Here's how the part is built. I have some questions about the finished solid (model axes, mm). A direction names the side the tool comes from. Coordinates: 2 decimals unless noted, no trailing zeros. Write each loop counter-clockwise with the first axis right and the second up, starting at its lowest first coordinate (ties: lowest second). Pieces come first, ordered by that corner, then holes.
```python
from build123d import *

# Parameters (mm, degrees)
BOSS_EXTRUDE1_DEPTH = 6.5


with BuildPart() as part:
    # Sketch1 → Boss-Extrude1 (new body)
    with BuildSketch(Plane.XY):
        with BuildLine():
            Line((9.441130989, 75.543158327), (10.978710332, 87.222232942))
            ThreePointArc((10.978710332, 87.222232942), (10.23623569, 89.872312951), (7.807292937, 91.166310537))
            ThreePointArc((7.807292937, 91.166310537), (0, 91.5), (-7.807292937, 91.166310537))
            ThreePointArc((-7.807292937, 91.166310537), (-10.23623569, 89.872312951), (-10.978710332, 87.222232942))
            Line((-10.978710332, 87.222232942), (-9.441130989, 75.543158327))
            ThreePointArc((-9.441130989, 75.543158327), (-8.278784327, 73.368560674), (-5.971073974, 72.5))
            Line((-5.971073974, 72.5), (5.971073974, 72.5))
            ThreePointArc((5.971073974, 72.5), (8.278784327, 73.368560674), (9.441130989, 75.543158327))
        make_face()
        with BuildLine():
            Line((-9.49154304, 87.418022231), (-7.953963697, 75.738947616))
            ThreePointArc((-7.953963697, 75.738947616), (-7.289765605, 74.496320385), (-5.971073974, 74))
            Line((-5.971073974, 74), (5.971073974, 74))
            ThreePointArc((5.971073974, 74), (7.289765605, 74.496320385), (7.953963697, 75.738947616))
            Line((7.953963697, 75.738947616), (9.49154304, 87.418022231))
            ThreePointArc((9.49154304, 87.418022231), (9.067271816, 88.932353664), (7.679304529, 89.671780856))
            ThreePointArc((7.679304529, 89.671780856), (0, 90), (-7.679304529, 89.671780856))
            ThreePointArc((-7.679304529, 89.671780856), (-9.067271816, 88.932353664), (-9.49154304, 87.418022231))
        make_face(mode=Mode.SUBTRACT)
    extrude(amount=BOSS_EXTRUDE1_DEPTH)


solid = part.part
```
1) Imagine slicing it at C-C on z = 1.25. Please give me the cut outline in (x, y), then the cut area to 3 significant figures.
Values follow:
outline: (-10.98, 87.22) - (-9.44, 75.54) arc R3.5 ccw to (-5.97, 72.5) - (5.97, 72.5) arc R3.5 ccw to (9.44, 75.54) - (10.98, 87.22) arc R3.5 ccw to (7.81, 91.17) arc R91.5 ccw to (-7.81, 91.17) arc R3.5 ccw to start; hole (-9.49, 87.42) - (-7.95, 75.74) arc R2 ccw to (-5.97, 74) - (5.97, 74) arc R2 ccw to (7.95, 75.74) - (9.49, 87.42) arc R2 ccw to (7.68, 89.67) arc R90 ccw to (-7.68, 89.67) arc R2 ccw to start
area: 102 mm2
2) We'd pull the mould along X, two halves only. Please class faces 3 (the face through (-0.1, 90.5, 6.5)), 4 (the face through (-10.211, 89.903, 3.204)), 5 (the face through (-8.734, 81.66, 3.204)), 6 (the face through (10.26, 89.84, 3.2)): pulls with the +X half, pulls with the -X half, needs draft (parallel to the pull), parting line crosses it, or undercut.
Values follow:
face 3: needs draft
face 4: pulls with the -X half
face 5: undercut
face 6: pulls with the +X half
3) Imagine slicing it at A-A on x = -6.5. Please give me the cut outline in (y, z).
Values follow:
outline: (72.54, 0) - (74.07, 0) - (74.07, 6.5) - (72.54, 6.5) - close; (89.76, 0) - (91.27, 0) - (91.27, 6.5) - (89.76, 6.5) - close
4) Will these pins go through, and if not, where does the flat tip stop? pin 1 (1.5 mm diameter, centred on x = 5, z = 5, fed in from +Y); pin 2 (1.5 mm diameter, centred on x = -6, y = 77.5, fed in from +Z); pin 3 (1.5 mm diameter, centred on y = 84, z = 1.5, fed in from -X); pin 4 (4 mm diameter, centred on x = -5, y = 89, fed in from -Z).
Values follow:
pin 1: stops at y = 91.4
pin 2: passes through
pin 3: stops at x = -10.65
pin 4: stops at z = 0
5) Imagine slicing it at B-B on y = 75. Please give me the cut outline in (x, z).
Values follow:
outline: (-9.33, 0) - (-7.7, 0) - (-7.7, 6.5) - (-9.33, 6.5) - close; (7.7, 0) - (9.33, 0) - (9.33, 6.5) - (7.7, 6.5) - close
6) I need wall thicknesses on probe 1 along X at (y, z) = (84.25, 4); probe 2 along X at (y, z) = (88.75, 4.25); probe 3 along Y at (x, z) = (-7.5, 5.5). Which ranges of each line are inside material? Lowest first, please.
Values follow:
probe 1: x = -10.59 to -9.07, 9.07 to 10.59
probe 2: x = -10.84 to -9.2, 9.2 to 10.84
probe 3: y = 72.85 to 74.71, 89.69 to 91.19
7) On a 3-axis mill with a long thin cutter (end or side, diameter ignored), from which of +Z, -Z, +X, -X, +Y, -Y can I reach the whole of each face in a straight line? I mean faces 1 (the face through (9.081, 88.915, 3.204)), 2 (the face through (8.252, 73.345, 3.204)). Say none if no direction works.
Values follow:
face 1: +Z, -Z
face 2: +Z, -Z, +X, -Y
